from build123d import *

# Parameters (mm, degrees)
SKETCH_2_W          = 70
SKETCH_2_H          = 75
SKETCH_2_W_2        = 60
SKETCH_2_H_2        = 65
EXTRUDE_1_DEPTH     = 2700
SKETCH_3_OUTSIDE_W  = 3242.39
SKETCH_3_OUTSIDE_H  = 617.39
CUT_EXTRUDE_1_DEPTH = 71


with BuildPart() as part:
    # Эскиз2 → Вытянуть-Тонкостенный1 (new body)
    with BuildSketch(Plane(origin=(0, 0, 0), x_dir=(0, 0, -1), z_dir=(1, 0, 0))):
        Rectangle(SKETCH_2_W, SKETCH_2_H)
        Rectangle(SKETCH_2_W_2, SKETCH_2_H_2, mode=Mode.SUBTRACT)
    extrude(amount=EXTRUDE_1_DEPTH)

    # Эскиз3 outside → Вырез-Вытянуть1 (cut, through all)
    with BuildSketch(Plane(origin=(0, 0, -35), x_dir=(-1, 0, 0), z_dir=(0, 0, -1))):
        with Locations((-1350, 0)):
            Rectangle(SKETCH_3_OUTSIDE_W, SKETCH_3_OUTSIDE_H)
        Polygon((-2700, -37.5), (-2625, 37.5), (-75, 37.5), (0, -37.5), align=None, mode=Mode.SUBTRACT)
    extrude(amount=-CUT_EXTRUDE_1_DEPTH, mode=Mode.SUBTRACT)


solid = part.part
Verification items for the finished model (mm, model axes). A direction names the side the tool comes from. Give positions to 0.01 mm unless a question says otherwise; leave off trailing zeros. Write each loop counter-clockwise with the first axis right and the second up, starting at its lowest first coordinate (ties: lowest second). Pieces come first, ordered by that corner, then holes. Notation, with made-up numbers: (-5.5, 68.25) -> (22.5, 68.25) arc R20 ccw to (22.5, 98.25) -> close; hole circle Ø6 at (54, 1). An arc over 180 degrees is marked (long way). Use CSV: the item, a comma, the result in double quotes.
(1) Sectioned sample at A-A (y = -13.5). Record the cut outline in (x, z), plus the area to 3 significant figures.
Derived:
outline,"(24, -35) -> (2676, -35) -> (2676, -30) -> (24, -30) -> close; (24, 30) -> (2676, 30) -> (2676, 35) -> (24, 35) -> close"
area,"26,500 mm^2"
(2) Sectioned sample at B-B (z = 7). Record the cut outline in (x, y).
Derived:
outline,"(0, -37.5) -> (2700, -37.5) -> (2695, -32.5) -> (5, -32.5) -> close; (70, 32.5) -> (2630, 32.5) -> (2625, 37.5) -> (75, 37.5) -> close"
(3) Sectioned sample at C-C (x = 1540). Record the cut outline in (y, z).
Derived:
outline,"(-37.5, -35) -> (37.5, -35) -> (37.5, 35) -> (-37.5, 35) -> close; hole (-32.5, -30) -> (32.5, -30) -> (32.5, 30) -> (-32.5, 30) -> close"
(4) Set-up check for faces 4 (the flat face through (1331, -32.5, 0)), 5 (the flat face through (1331, -37.5, 0)): record each of +Z, -Z, +X, -X, +Y, -Y from which the full face is reachable in a straight line by a thin tool's end or side.
Derived:
face 4,"+X, -X"
face 5,"+Z, -Z, +X, -X, -Y"
(5) Go/stop test with a flat-tipped pin: pin 1 (8 mm diameter, centred on y = 3, z = -25, fed in from +X). Record where the tip stops, or that it passes through.
Derived:
pin 1,"passes through"
(6) Release check for a two-part mould opening along Z. For faces 1 (the flat face through (1331, 0, 30)), 2 (the flat face through (1332, 37.5, 0)), 3 (the flat face through (1331, -1, 35)) record: +Z half, -Z half, draft (parallel to the pull), parting line (faces both ways), or undercut.
Derived:
face 1,"undercut"
face 2,"draft"
face 3,"+Z half"
(7) Material ranges on L1, parallel to Y at x = 759.5, z = 14; L2, parallel to Z at x = 300, y = -31; L3, parallel to X at y = -26, z = -31, recorded low to high.
Derived:
L1,"y = -37.5 to -32.5, 32.5 to 37.5"
L2,"z = -35 to -30, 30 to 35"
L3,"x = 11.5 to 2688.5"
